Here's the drawing with two shaded views (mm, measured from the low corner). I have some questions. Coordinates: 2 decimals unless noted, no trailing zeros. Write each loop counter-clockwise with the first axis right and the second up, starting at its lowest first coordinate (ties: lowest second). Pieces come first, ordered by that corner, then holes. Notation, with made-up numbers: (-1.5, 54.5) -> (27.5, 54.5) arc R25 cw to (27.5, 91.5) -> close; hole circle Ø6 at (59.5, 67.5). An arc over 180 degrees is marked (long way). Answer in a Markdown table with one row per item. Add a question column.
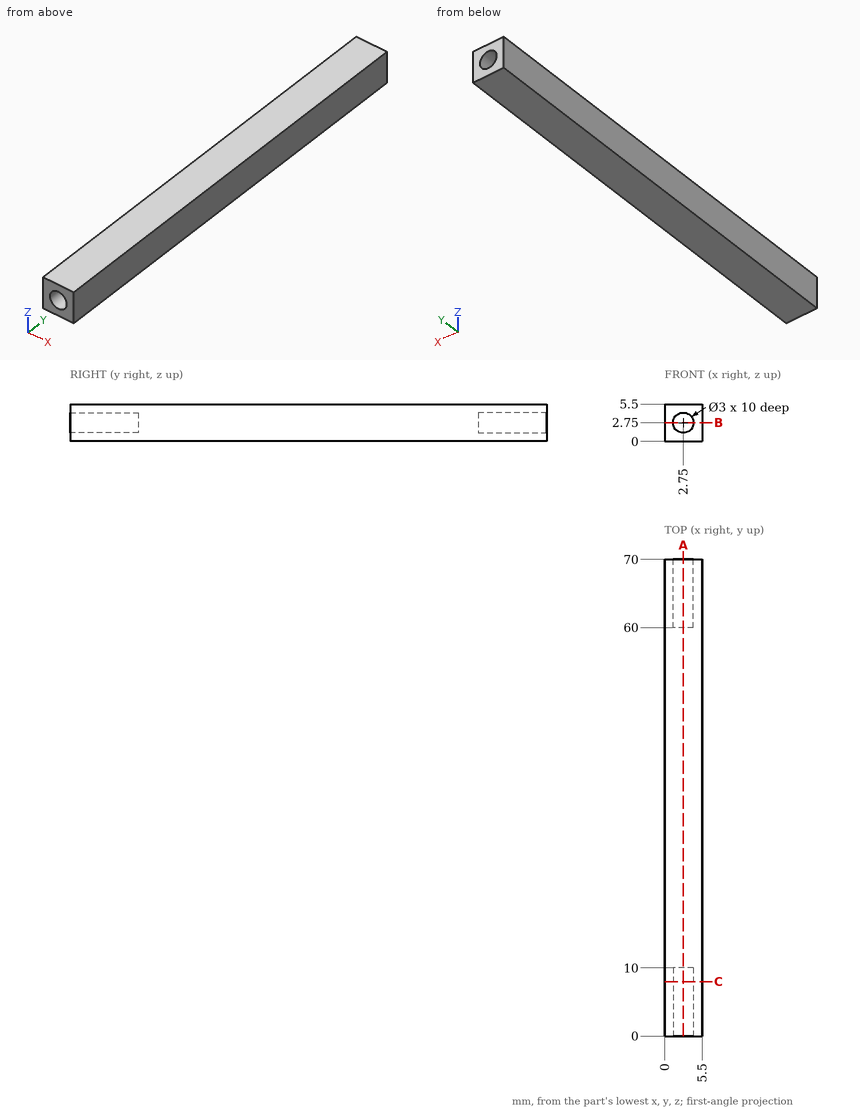
Q1. I'm going to push a flat-ended pin straight in: P1, Ø2, axis at x = 2.5, z = 3, coming from the +Y side. Where does the tip first touch, or does it pass through?
Q2. Imagine slicing it at A-A on x = 2.75. Please give me the cut outline in (y, z), plus the area to 3 significant figures.
Q3. Imagine slicing it at B-B on z = 2.75. Please give me the cut outline in (x, y).
Q4. Imagine slicing it at C-C on y = 8. Please give me the cut outline in (x, z), plus the area to 3 significant figures.
Q5. I need wall thicknesses on line 1 (X direction, y = 3, z = 2.75); line 2 (Y direction, x = 2.75, z = 3.3); line 3 (X direction, y = 64.5, z = 1.9). Which ranges of each line are inside material? Lowest first, please. Write a range as [from, to].
Result sheet:
| question | item | result |
|---|---|---|
| 1 | P1 | stops at y = 60 |
| 2 | outline | (0, 0) -> (70, 0) -> (70, 1.25) -> (60, 1.25) -> (60, 4.25) -> (70, 4.25) -> (70, 5.5) -> (0, 5.5) -> (0, 4.25) -> (10, 4.25) -> (10, 1.25) -> (0, 1.25) -> close |
| 2 | area | 325 mm^2 |
| 3 | outline | (0, 0) -> (1.25, 0) -> (1.25, 10) -> (4.25, 10) -> (4.25, 0) -> (5.5, 0) -> (5.5, 70) -> (4.25, 70) -> (4.25, 60) -> (1.25, 60) -> (1.25, 70) -> (0, 70) -> close |
| 4 | outline | (0, 0) -> (5.5, 0) -> (5.5, 5.5) -> (0, 5.5) -> close; hole circle Ø3 at (2.75, 2.75) |
| 4 | area | 23.2 mm^2 |
| 5 | line 1 | x = [0, 1.25], [4.25, 5.5] |
| 5 | line 2 | y = [10, 60] |
| 5 | line 3 | x = [0, 1.51], [3.99, 5.5] |
